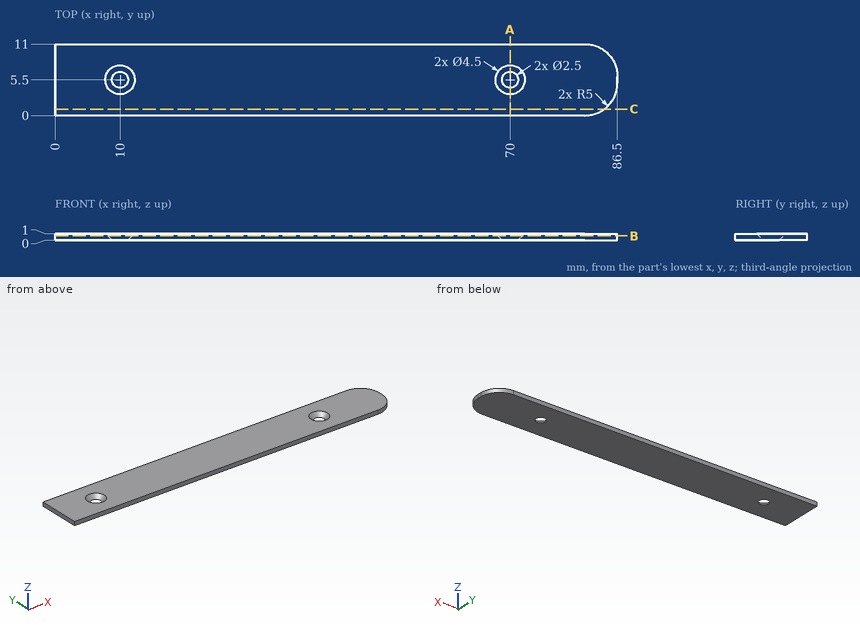
Here's the drawing with two shaded views (mm, measured from the low corner). I have some questions. Give positions to 0.01 mm unless a question says otherwise; leave off trailing zeros. Write each loop counter-clockwise with the first axis right and the second up, starting at its lowest first coordinate (ties: lowest second). Pieces come first, ordered by that corner, then holes. Notation, with made-up numbers: (-1, -28) -> (44, -28) arc R20 cw to (44, -2) -> close; hole circle Ø9 at (75, -31). An arc over 180 degrees is marked (long way). Use one line per item in the form item = value. Start each with the question number.
1. Imagine slicing it at C-C on y = 1. List the corners of the cut face in (x, z) for me, plus the area to 3 significant figures.
2. If I drill on L1, parallel to X at y = 6.25, z = 0.85; L2, parallel to Y at x = 70.5, z = 0.95; L3, parallel to X at y = 9.25, z = 0.2, over which ranges is the centre line in solid material (lowest first)?
3. Imagine slicing it at B-B on z = 0.65. List the corners of the cut face in (x, y) for me.
4. Imagine slicing it at A-A on x = 70. List the corners of the cut face in (y, z) for me.
Entries:
q1.outline = (0, 0) -> (84.5, 0) -> (84.5, 1) -> (0, 1) -> close
q1.area = 84.5 mm²
q2.L1 = 0 to 8.04, 11.96 to 68.04, 71.96 to 86.49
q2.L2 = 0 to 3.36, 7.64 to 11
q2.L3 = 0 to 85.3
q3.outline = (0, 0) -> (81.5, 0) arc R5 ccw to (86.5, 5) -> (86.5, 6) arc R5 ccw to (81.5, 11) -> (0, 11) -> close; hole circle Ø3.8 at (10, 5.5); hole circle Ø3.8 at (70, 5.5)
q4.outline = (0, 0) -> (4.25, 0) -> (3.25, 1) -> (0, 1) -> close; (6.75, 0) -> (11, 0) -> (11, 1) -> (7.75, 1) -> close
